Source: CAD feature listing. Evaluate the final solid. Frame: model axes, mm. A direction names the side the tool comes from. Give positions to 0.01 mm unless a question says otherwise; leave off trailing zeros. Order: outer loops, then holes, each group sorted by start corner. A loop starts at its lowest first (then second) coordinate and runs counter-clockwise, first axis right, second up. Notation, with made-up numbers: (35.25, 7) -> (83.25, 7) arc R5 ccw to (83.25, 12) -> close; hole circle Ø11 at (74, -1.75). An arc over 180 degrees is marked (long way). Use CSV: the item, a comma, the result in double quotes.
```python
from build123d import *

# Parameters (mm, degrees)
F1_DEPTH       = 3.175
F3_D           = 4.7625
F3_DEPTH       = 19.05
F3_CSINK_D     = 5.5372
F3_CSINK_ANGLE = 135
F3_TIP         = 1.4307993491


with BuildPart() as f1:
    # F0 (on Front) → F1 (new body, symmetric)
    with BuildSketch(Plane.XZ):
        Polygon((-57.15, 20.6375), (-63.5, 20.6375), (-63.5, -20.6375), (-57.15, -20.6375), (-57.15, -15.875), (0, -15.875), (0, 15.875), (-57.15, 15.875), align=None)
    extrude(amount=F1_DEPTH, both=True)

    # F3
    with Locations(Plane.YZ):
        with Locations((0, 11.1125), (0, -6.35)):
            CounterSinkHole(F3_D / 2, F3_CSINK_D / 2, depth=F3_DEPTH, counter_sink_angle=F3_CSINK_ANGLE)
            with Locations((0, 0, -(F3_DEPTH + F3_TIP / 2))):  # 118° drill point
                Cone(0, F3_D / 2, F3_TIP, mode=Mode.SUBTRACT)


solid = f1.part
```
1. Section query B-B on x = -9. Count the separate pieces of the cut face and the enclosed holes in it, plus the area to 3 significant figures.
Answer below:
separate pieces,"1"
enclosed holes,"2"
area,"166 mm²"
2. Ray query, line 1 along Z through (x, y) = (-10, 0) (3 decimals); line 2 along Y through (x, z) = (-9.25, -6.35) (3 decimals); line 3 along Z through (x, y) = (-17, -2) (3 decimals). Return the intervals inside material, ascending.
Answer below:
line 1,"z = -15.875 to -8.731, -3.969 to 8.731, 13.494 to 15.875"
line 2,"y = -3.175 to -2.381, 2.381 to 3.175"
line 3,"z = -15.875 to -7.642, -5.058 to 9.82, 12.405 to 15.875"
3. Access query for faces 1 (the flat face through (-60, 0, -20.638)), 2 (the flat face through (-29, 0, -15.875)), 3 (the cylindrical face through (-9.737, 0.31, 13.473)), 4 (the flat face through (-57.15, 0, 18)), 5 (the flat face through (-32, 3.175, 0)). Directions: +Z, -Z, +X, -X, +Y, -Y. A direction counts if a zero-diameter tool reaches every point of the face in a straight line with its end or side. Return the directions, or none.
Answer below:
face 1,"-Z, +X, -X, +Y, -Y"
face 2,"-Z, +X, +Y, -Y"
face 3,"+X"
face 4,"+Z, +X, +Y, -Y"
face 5,"+Z, -Z, +X, -X, +Y"
4. Section query C-C on x = -44.5. Return loops of the section in (y, z) (3 decimals), plus the area to 3 significant figures.
Answer below:
outline,"(-3.175, -15.875) -> (3.175, -15.875) -> (3.175, 15.875) -> (-3.175, 15.875) -> close"
area,"202 mm²"
5. Section query A-A on z = 17. Return loops of the section in (x, y) (3 decimals).
Answer below:
outline,"(-63.5, -3.175) -> (-57.15, -3.175) -> (-57.15, 3.175) -> (-63.5, 3.175) -> close"
6. Mould query, pull axis Y, two halves, no side actions, for faces 6 (the flat face through (-57.15, 0, -18)), 7 (the flat face through (-32, -3.175, 0)), 8 (the conical face through (-20.23, 0.19, -6.72)). Classes: released by +Y, released by -Y, zero draft, split by the parting line, or undercut.
Answer below:
face 6,"zero draft"
face 7,"released by -Y"
face 8,"undercut"
